```python
from build123d import *

# Parameters (mm, degrees)
CUT_EXTRUDE1_DEPTH      = 26.4000001
CUT_EXTRUDE1_DEPTH_BACK = 1.0000001


with BuildPart() as part:
    # Sketch2 → Loft1 section 0
    with BuildSketch(Plane(origin=(0, 0, 0), x_dir=(1, 0, 0), z_dir=(0, 1, 0))):
        with BuildLine():
            Line((-4.71851035, 11.790914302), (-2.1, 31.68047506))
            ThreePointArc((-2.1, 31.68047506), (0, 31.75), (2.1, 31.68047506))
            Line((2.1, 31.68047506), (4.71851035, 11.790914302))
            ThreePointArc((4.71851035, 11.790914302), (8.980256121, 8.980256121), (11.790914302, 4.71851035))
            Line((11.790914302, 4.71851035), (31.68047506, 2.1))
            ThreePointArc((31.68047506, 2.1), (31.75, 0), (31.68047506, -2.1))
            Line((31.68047506, -2.1), (11.790914302, -4.71851035))
            ThreePointArc((11.790914302, -4.71851035), (8.980256121, -8.980256121), (4.71851035, -11.790914302))
            Line((4.71851035, -11.790914302), (2.1, -31.68047506))
            ThreePointArc((2.1, -31.68047506), (0, -31.75), (-2.1, -31.68047506))
            Line((-2.1, -31.68047506), (-4.71851035, -11.790914302))
            ThreePointArc((-4.71851035, -11.790914302), (-8.980256121, -8.980256121), (-11.790914302, -4.71851035))
            Line((-11.790914302, -4.71851035), (-31.68047506, -2.1))
            ThreePointArc((-31.68047506, -2.1), (-31.75, 0), (-31.68047506, 2.1))
            Line((-31.68047506, 2.1), (-11.790914302, 4.71851035))
            ThreePointArc((-11.790914302, 4.71851035), (-8.980256121, 8.980256121), (-4.71851035, 11.790914302))
        make_face()
    # Sketch5 → Loft1 section 1
    with BuildSketch(Plane(origin=(0, 25.4, 0), x_dir=(1, 0, 0), z_dir=(0, 1, 0))):
        with BuildLine():
            Line((-4.13090623, 4.822666661), (-1.85, 22.147869536))
            ThreePointArc((-1.85, 22.147869536), (0, 22.225), (1.85, 22.147869536))
            Line((1.85, 22.147869536), (4.13090623, 4.822666661))
            ThreePointArc((4.13090623, 4.822666661), (4.490128061, 4.490128061), (4.822666661, 4.13090623))
            Line((4.822666661, 4.13090623), (22.147869536, 1.85))
            ThreePointArc((22.147869536, 1.85), (22.225, 0), (22.147869536, -1.85))
            Line((22.147869536, -1.85), (4.822666661, -4.13090623))
            ThreePointArc((4.822666661, -4.13090623), (4.490128061, -4.490128061), (4.13090623, -4.822666661))
            Line((4.13090623, -4.822666661), (1.85, -22.147869536))
            ThreePointArc((1.85, -22.147869536), (0, -22.225), (-1.85, -22.147869536))
            Line((-1.85, -22.147869536), (-4.13090623, -4.822666661))
            ThreePointArc((-4.13090623, -4.822666661), (-4.490128061, -4.490128061), (-4.822666661, -4.13090623))
            Line((-4.822666661, -4.13090623), (-22.147869536, -1.85))
            ThreePointArc((-22.147869536, -1.85), (-22.225, 0), (-22.147869536, 1.85))
            Line((-22.147869536, 1.85), (-4.822666661, 4.13090623))
            ThreePointArc((-4.822666661, 4.13090623), (-4.490128061, 4.490128061), (-4.13090623, 4.822666661))
        make_face()
    loft()

    # Sketch2<3> → Cut-Extrude1 (cut, two sides)
    with BuildSketch(Plane(origin=(0, 0, 0), x_dir=(1, 0, 0), z_dir=(0, 1, 0))) as cut_extrude1_sk:
        with BuildLine():
            ThreePointArc((2.236067977, 2), (0, -3), (-2.236067977, 2))
            Line((-2.236067977, 2), (2.236067977, 2))
        make_face()
    extrude(amount=CUT_EXTRUDE1_DEPTH, mode=Mode.SUBTRACT)
    extrude(cut_extrude1_sk.sketch, amount=-CUT_EXTRUDE1_DEPTH_BACK, mode=Mode.SUBTRACT)


solid = part.part
```
Model file for the job. Use its own axes, mm. A direction names the side the tool comes from. Round coordinates to 2 decimals unless told otherwise and drop trailing zeros. Use one line per item in the form item = value.
Item 1: Pull direction Z, two halves, no side cores. Call faces 1 (the face through (-3.2, 25.4, 0.4)), 2 (the face through (0, 13, 3)): released by +Z, released by -Z, zero draft, split by the parting line, or undercut.
Returned:
face_1 = zero draft
face_2 = undercut
Item 2: Drill centre lines: line 1 (X direction, y = 12.25, z = 0); line 2 (X direction, y = 19.5, z = 0); line 3 (Z direction, x = 0, y = 19.5). Where is each one in solid material? Low to high.
Returned:
line_1 = -27.16 to -3, 3 to 27.16
line_2 = -24.44 to -3, 3 to 24.44
line_3 = -24.44 to -2, 3 to 24.44
Item 3: Flat gauge pins, fed straight in: pin 1 Ø6 at (y, z) = (18.5, -11.5) entering from -X; pin 2 Ø3.5 at (x, y) = (-1, 6.5) entering from +Z; pin 3 Ø6 at (y, z) = (6, 15) entering from -X. Where does each tip first touch, or does it go through?
Returned:
pin_1 = -4.09
pin_2 = 29.95
pin_3 = -4.37
Item 4: Tool access for faces 3 (the face through (0, 13, -2)), 4 (the face through (3, 0, 2)): list every direction of +Z, -Z, +X, -X, +Y, -Y with a clear straight run to the whole face (end or side of a thin tool).
Returned:
face_3 = +Y, -Y
face_4 = +Z, -Z, +X, -X, -Y
